The listing builds one solid part. Answer for the finished solid, in the listing's coordinates (mm). Face numbers are marked on the shaded views. A direction names the side the tool comes from. Coordinates: 2 decimals unless noted, no trailing zeros. Loops run counter-clockwise (first coordinate to the right, second up) from the corner with the lowest first, then second, coordinate; pieces in that order, holes last. Notation, with made-up numbers: M -20.75,-8.75 L -4.75,-8.75 A13 cw -4.75,6.25 Z; hole C 86,-9 d11. An arc over 180 degrees is marked long. Return JSON: item names as keys, results as strings. Group by question number.
1. Section D-D (z = 49.5) is taken. Write down the section's boundary in (x, y).
2. Given P1, Ø12, axis at y = 41.5, z = -18, coming from the +X side; P2, Ø1.5, axis at y = 169, z = 12.5, coming from the -X side; P3, Ø18.5, axis at x = -25.4, z = -25.4, coming from the +Y side; P4, Ø10, axis at y = 76.5, z = -25, coming from the +X side, each flat-ended and moving along its own axis, determine where each tip first touches the part or whether it passes through.
3. The mould has two halves that part along X. Classify the marked faces 1, 2 and 3: pulls with the +X half, pulls with the -X half, needs draft (parallel to the pull), parting line crosses it, or undercut.
4. Section C-C (x = 28.5) is taken. Write down the section's boundary in (y, z).
5. Straight lines are drawn through the part: L1, parallel to X at y = 157, z = 25.5; L2, parallel to X at y = 44, z = 21.5; L3, parallel to Z at x = -35, y = 136. For each, find the intervals that lie inside material, in ascending order. Write a range as from..to.
6. Which of the six approach directions +Z, -Z, +X, -X, +Y, -Y give full straight-line access (tool end or side, diameter ignored) to the marked faces 4, 5 and 6?
7. Section A-A (y = 173) is taken. Write down the section's boundary in (x, z) (1 decimal).
8. Section B-B (z = -25.4) is taken. Write down the section's boundary in (x, y).
```python
from build123d import *

# Parameters (mm, degrees)
SKETCH1_R           = 91.7575
BOSS_EXTRUDE1_DEPTH = 228.6
SKETCH2_R           = 48.26
SKETCH2_R_2         = 38.1
CUT_EXTRUDE1_DEPTH  = 50.8
SKETCH4_R           = 15.24
CUT_EXTRUDE2_DEPTH  = 177.8
SKETCH5_R           = 15.24
CUT_EXTRUDE3_DEPTH  = 177.8
SKETCH6_R           = 38.1
CUT_EXTRUDE9_DEPTH  = 50.8


with BuildPart() as part:
    # Sketch1 → Boss-Extrude1 (new body)
    with BuildSketch(Plane(origin=(0, 0, 0), x_dir=(1, 0, 0), z_dir=(0, 1, 0))):
        with Locations(Location((0, 0, 0), (0, 0, 270))):
            Circle(SKETCH1_R)
    extrude(amount=BOSS_EXTRUDE1_DEPTH)

    # Sketch2 → Cut-Extrude1 (cut)
    with BuildSketch(Plane(origin=(0, 228.6, 0), x_dir=(1, 0, 0), z_dir=(0, 1, 0))):
        with Locations((-34.29, 34.29)):
            Circle(SKETCH2_R)
        with Locations(Location((34.29, -34.29, 0), (0, 0, 270))):
            Circle(SKETCH2_R_2)
    extrude(amount=-CUT_EXTRUDE1_DEPTH, mode=Mode.SUBTRACT)

    # Sketch4 → Cut-Extrude2 (cut)
    with BuildSketch(Plane(origin=(0, 228.6, 0), x_dir=(1, 0, 0), z_dir=(0, 1, 0))):
        with Locations(Location((25.4, 25.4, 0), (0, 0, 270))):
            Circle(SKETCH4_R)
        with Locations(Location((-25.4, -25.4, 0), (0, 0, 270))):
            Circle(SKETCH4_R)
    extrude(amount=-CUT_EXTRUDE2_DEPTH, mode=Mode.SUBTRACT)

    # Sketch5 → Cut-Extrude3 (cut)
    with BuildSketch(Plane.XZ):
        with Locations(Location((-25.4, -25.4, 0), (0, 0, 270))):
            Circle(SKETCH5_R)
        with Locations(Location((25.4, 25.4, 0), (0, 0, 270))):
            Circle(SKETCH5_R)
    extrude(amount=-CUT_EXTRUDE3_DEPTH, mode=Mode.SUBTRACT)

    # Sketch6 → Cut-Extrude9 (cut)
    with BuildSketch(Plane.XZ):
        with Locations(Location((-34.29, 34.29, 0), (0, 0, 270))):
            Circle(SKETCH6_R)
        with Locations(Location((34.29, -34.29, 0), (0, 0, 270))):
            Circle(SKETCH6_R)
    extrude(amount=-CUT_EXTRUDE9_DEPTH, mode=Mode.SUBTRACT)


solid = part.part
```
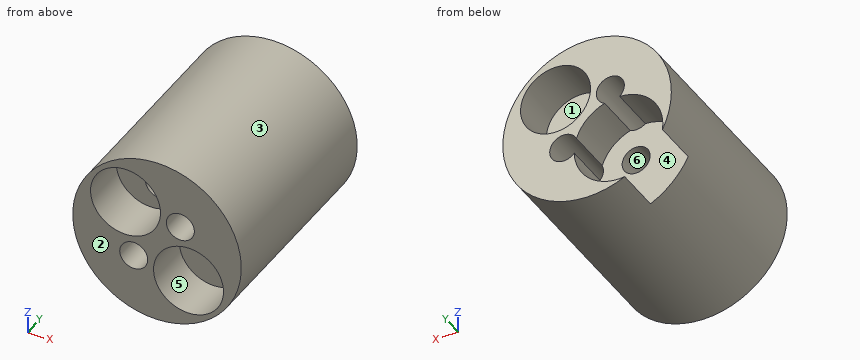
Worked out:
{
 "1": {"outline": "M -77.26,0 L -69.22,0 L -69.22,50.8 L 0.64,50.8 L 0.64,0 L 77.26,0 L 77.26,228.6 L 69.22,228.6 L 69.22,177.8 L -0.64,177.8 L -0.64,228.6 L -77.26,228.6 Z"},
 "2": {"P1": "x = 90.97", "P2": "x = -91", "P3": "through", "P4": "x = 89.55"},
 "3": {"face 1": "undercut", "face 2": "needs draft", "face 3": "parting line crosses it"},
 "4": {"outline": "M 0,-87.22 L 228.6,-87.22 L 228.6,-40.32 L 50.8,-40.32 L 50.8,-71.95 L 0,-71.95 Z; M 0,3.37 L 50.8,3.37 L 50.8,-10.48 L 228.6,-10.48 L 228.6,-3.37 L 177.8,-3.37 L 177.8,10.48 L 0,10.48 Z; M 0,40.32 L 177.8,40.32 L 177.8,71.95 L 228.6,71.95 L 228.6,87.22 L 0,87.22 Z"},
 "5": {"L1": "-88.14..-40.64, -10.16..10.16, 40.64..88.14", "L2": "-89.2..-70.18, 1.6..10.67, 40.13..89.2", "L3": "-84.82..-37.24, -13.56..13.56, 37.24..84.82"},
 "6": {"face 4": "+Y", "face 5": "-Y", "face 6": "+Y, -Y"},
 "7": {"outline": "C 0,0 d183.5; hole C -25.4,-25.4 d30.5; hole C -25.4,25.4 d30.5; hole C 25.4,-25.4 d30.5; hole C 25.4,25.4 d30.5"},
 "8": {"outline": "M -88.17,0 L -40.64,0 L -40.64,177.8 L -81.72,177.8 L -81.72,228.6 L -88.17,228.6 Z; M -10.16,0 L -2.76,0 L -2.76,50.8 L 10.16,50.8 L 10.16,177.8 L -10.16,177.8 Z; M 40.64,50.8 L 71.34,50.8 L 71.34,0 L 88.17,0 L 88.17,228.6 L 40.64,228.6 Z"}
}
